Design review of the part shown in the three views and the two pictorial views. Dimensions are in mm from the part's minimum x, y and z. Give positions to 0.01 mm unless a question says otherwise; leave off trailing zeros. Order: outer loops, then holes, each group sorted by start corner. A loop starts at its lowest first (then second) coordinate and runs counter-clockwise, first axis right, second up. Notation, with made-up numbers: (26.5, 22.25) - (78.5, 22.25) arc R19 cw to (78.5, 55.25) - close; hole circle Ø6 at (72, 71). An arc over 180 degrees is marked (long way). Put each result on its own line as item: value.
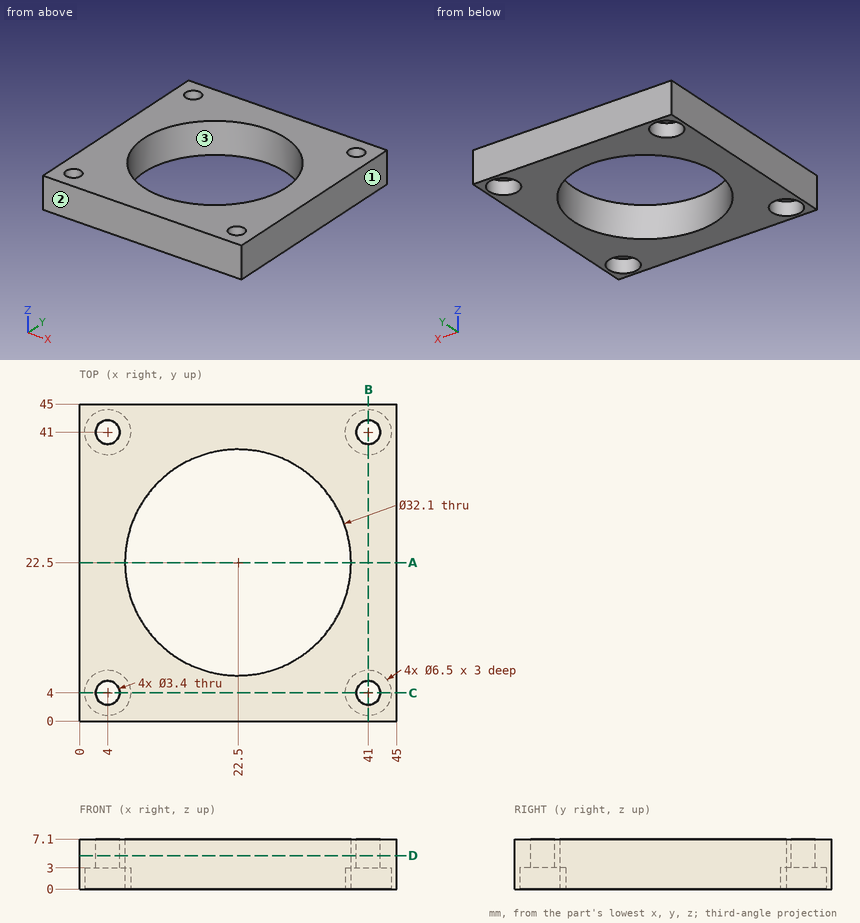
(1) Take a section at D-D, the plane z = 4.75. Write out the cut boundary in (x, y).
The answers:
outline: (0, 0) - (45, 0) - (45, 45) - (0, 45) - close; hole circle Ø3.4 at (4, 4); hole circle Ø3.4 at (4, 41); hole circle Ø32.1 at (22.5, 22.5); hole circle Ø3.4 at (41, 4); hole circle Ø3.4 at (41, 41)
(2) Clearance check with flat-ended pins moving along their axes: pin 1 Ø3 at (x, y) = (4, 4) entering from -Z; pin 2 Ø5 at (x, y) = (4, 41) entering from -Z. State where each tip first meets the part, or that it passes through.
The answers:
pin 1: through
pin 2: z = 3
(3) Take a section at B-B, the plane x = 41. Write out the cut boundary in (y, z), then the cut area to 3 significant figures.
The answers:
outline: (0, 0) - (0.75, 0) - (0.75, 3) - (2.3, 3) - (2.3, 7.1) - (0, 7.1) - close; (5.7, 3) - (7.25, 3) - (7.25, 0) - (37.75, 0) - (37.75, 3) - (39.3, 3) - (39.3, 7.1) - (5.7, 7.1) - close; (42.7, 3) - (44.25, 3) - (44.25, 0) - (45, 0) - (45, 7.1) - (42.7, 7.1) - close
area: 253 mm^2
(4) The part is to be moulded in two halves that separate along X. For the marked faces 1, 2 and 3, say which applies: pulls with the +X half, pulls with the -X half, needs draft (parallel to the pull), parting line crosses it, or undercut.
The answers:
face 1: pulls with the +X half
face 2: needs draft
face 3: undercut
(5) Wall thickness on L1, parallel to Y at x = 4, z = 0.6; L2, parallel to Y at x = 4, z = 6.05: over which ranges is each line inside the solid? List them lowest first.
The answers:
L1: 0 to 0.75, 7.25 to 37.75, 44.25 to 45
L2: 0 to 2.3, 5.7 to 39.3, 42.7 to 45
(6) Take a section at A-A, the plane y = 22.5. Write out the cut boundary in (x, z).
The answers:
outline: (0, 0) - (6.45, 0) - (6.45, 7.1) - (0, 7.1) - close; (38.55, 0) - (45, 0) - (45, 7.1) - (38.55, 7.1) - close
